The figure shows three views and two pictorial views of one solid part (mm, origin at its lowest corner). Answer the questions. A direction names the side the tool comes from. Give positions to 0.01 mm unless a question says otherwise; leave off trailing zeros. Order: outer loops, then holes, each group sorted by start corner. A loop starts at its lowest first (then second) coordinate and runs counter-clockwise, first axis right, second up. Notation, with made-up numbers: M 83,16.25 L 135,16.25 A12 ccw 135,32.25 Z; hole C 73,47.5 d1. An arc over 180 degrees is marked long. Write item = value, one per line. Start each with the question number.
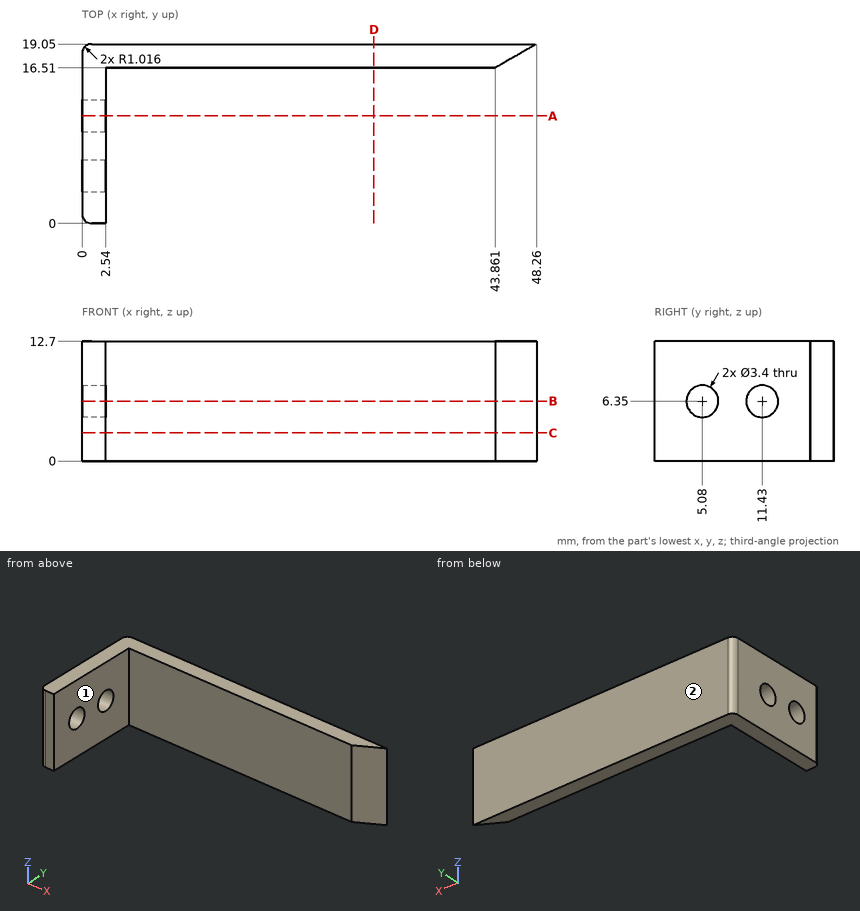
1) Find the intervals of material crossed by probe 1 along Y at (x, z) = (1.4, 6.35); probe 2 along X at (y, z) = (1.75, 4); probe 3 along Y at (x, z) = (0.6, 6.35), in increasing order. Write a range as [from, to].
2) Find section B-B on z = 6.35. Determine the outline of the cut face in (x, y).
3) Find section C-C on z = 3. Determine the outline of the cut face in (x, y).
4) Find section D-D on x = 31. Determine the outline of the cut face in (y, z).
5) For the marked faces 1 and 2, determine the directions among +Z, -Z, +X, -X, +Y, -Y from which every point of the face is accessible in a straight line to the end or side of a thin tool.
6) Find section A-A on y = 11.43. Determine the outline of the cut face in (x, z).
7) Each of these flat-tipped pins is pushed along its axis until it touches: P1, Ø4.5, axis at y = 11.43, z = 6.35, coming from the +X side; P2, Ø4, axis at x = 31.5, z = 6, coming from the -Y side. Where does it stop, or does it pass through?
Numbers:
q1.probe_1 = [0, 3.38], [6.78, 9.73], [13.13, 19.05]
q1.probe_2 = [0, 2.54]
q1.probe_3 = [0.09, 3.38], [6.78, 9.73], [13.13, 18.96]
q2.outline = M 0,1.02 A1.02 ccw 1.02,0 L 2.54,0 L 2.54,3.38 L 0,3.38 Z; M 0,6.78 L 2.54,6.78 L 2.54,9.73 L 0,9.73 Z; M 0,13.13 L 2.54,13.13 L 2.54,16.51 L 43.86,16.51 L 48.26,19.05 L 1.02,19.05 A1.02 ccw 0,18.03 Z
q3.outline = M 0,1.02 A1.02 ccw 1.02,0 L 2.54,0 L 2.54,16.51 L 43.86,16.51 L 48.26,19.05 L 1.02,19.05 A1.02 ccw 0,18.03 Z
q4.outline = M 16.51,0 L 19.05,0 L 19.05,12.7 L 16.51,12.7 Z
q5.face_1 = +Z, -Z, +X, -Y
q5.face_2 = +Z, -Z, +X, -X, +Y
q6.outline = M 0,0 L 2.54,0 L 2.54,4.65 L 0,4.65 Z; M 0,8.05 L 2.54,8.05 L 2.54,12.7 L 0,12.7 Z
q7.P1 = 2.54
q7.P2 = 16.51
